```python
from build123d import *

# Parameters (mm, degrees)
F1_DEPTH = 25
F2_DEPTH = 7.5
F3_DEPTH = 12.5
F4_R     = 10
F5_F1_R  = 2
F5_F2_R  = 2
F6_R     = 3.5
F7_DEPTH = 15
F8_R     = 1.99999


# Not quite as in the source:
# - a fillet or chamfer is up to 0.001 mm smaller than in the source, because OpenCascade refuses the exact size


with BuildPart() as f1:
    # F0 (on Top) → F1 (new body, symmetric)
    with BuildSketch(Plane.XY):
        Polygon((-32.5, 5), (-50, 5), (-50, -5), (0, -5), (0, 5), (-17.5, 5), align=None)
    extrude(amount=F1_DEPTH, both=True)

    # F0 (on Top) → F2 (join, symmetric)
    with BuildSketch(Plane.XY):
        with BuildLine():
            Line((-32.5, 28), (-32.5, 5))
            Line((-32.5, 5), (-17.5, 5))
            Line((-17.5, 5), (-17.5, 21))
            ThreePointArc((-17.5, 21), (-14.8639610307, 27.3639610307), (-8.5, 30))
            Line((-8.5, 30), (10, 30))
            Line((10, 30), (10, 37))
            Line((10, 37), (-23.5, 37))
            ThreePointArc((-23.5, 37), (-29.8639610307, 34.3639610307), (-32.5, 28))
        make_face()
    extrude(amount=F2_DEPTH, both=True)

    # F0 (on Top) → F3 (join, symmetric)
    with BuildSketch(Plane.XY):
        Polygon((10, 41), (10, 37), (10, 30), (10, 26), (30, 26), (30, 41), align=None)
    extrude(amount=F3_DEPTH, both=True)

    # F4
    f4_edges = [f1.edges().sort_by_distance(p)[0] for p in [
        (-50, 0, 25),
        (0, 0, 25),
        (0, 0, -25),
        (-50, 0, -25),
    ]]
    fillet(f4_edges, radius=F4_R)

    # F5: fillet of radius 2 on 26 edges, made by hand

    # F5_f1
    f5_f1_edges = [f1.edges().sort_by_distance(p)[0] for p in [
        (0.75, 30, 7.5),
        (-6.75, 37, 7.5),
        (-29.8639610307, 34.3639610307, 7.5),
        (-32.5, 16.5, 7.5),
        (-17.5, 13, 7.5),
        (-14.8639610307, 27.3639610307, 7.5),
        (0.75, 30, -7.5),
        (-6.75, 37, -7.5),
        (-29.8639610307, 34.3639610307, -7.5),
        (-32.5, 16.5, -7.5),
        (-17.5, 13, -7.5),
        (-14.8639610307, 27.3639610307, -7.5),
        (-50, 5, 0),
        (-47.0710678119, 5, -22.0710678119),
        (-47.0710678119, 5, 22.0710678119),
        (-25, 5, -25),
        (-25, 5, 25),
        (-2.9289321881, 5, -22.0710678119),
        (-2.9289321881, 5, 22.0710678119),
        (0, 5, 0),
    ]]
    fillet(f5_f1_edges, radius=F5_F1_R)

    # F5_f2
    f5_f2_edges = [f1.edges().sort_by_distance(p)[0] for p in [
        (10, 33.5, 7.5),
        (-25, 5, 7.5),
        (10, 33.5, -7.5),
        (-25, 5, -7.5),
        (-17.5, 5, 0),
        (-32.5, 5, 0),
        (-31.9142135624, 5, -6.9142135624),
        (-31.9142135624, 5, 6.9142135624),
        (-18.0857864376, 5, 6.9142135624),
        (-18.0857864376, 5, -6.9142135624),
        (10, 30.5857864376, -6.9142135624),
        (10, 36.4142135624, -6.9142135624),
        (10, 30.5857864376, 6.9142135624),
        (10, 36.4142135624, 6.9142135624),
    ]]
    fillet(f5_f2_edges, radius=F5_F2_R)

    # F6 (on face) → F7 (cut, through all)
    with BuildSketch(Plane(origin=(0, 41, 0), x_dir=(-1, 0, 0), z_dir=(0, 1, 0))):
        with Locations((-20, 0)):
            Circle(F6_R)
    extrude(amount=-F7_DEPTH, mode=Mode.SUBTRACT)

    # F8 (radius 2 in the source; OpenCascade refuses exactly that, so slightly less here)
    f8_edges = [f1.edges().sort_by_distance(p)[0] for p in [
        (10, 33.5, -12.5),
        (20, 26, -12.5),
        (30, 33.5, -12.5),
        (20, 41, -12.5),
        (10, 33.5, 12.5),
        (20, 26, 12.5),
        (30, 33.5, 12.5),
        (20, 41, 12.5),
        (30, 41, 0),
        (30, 26, 0),
        (10, 41, 0),
        (10, 26, 0),
    ]]
    fillet(f8_edges, radius=F8_R)


solid = f1.part
```
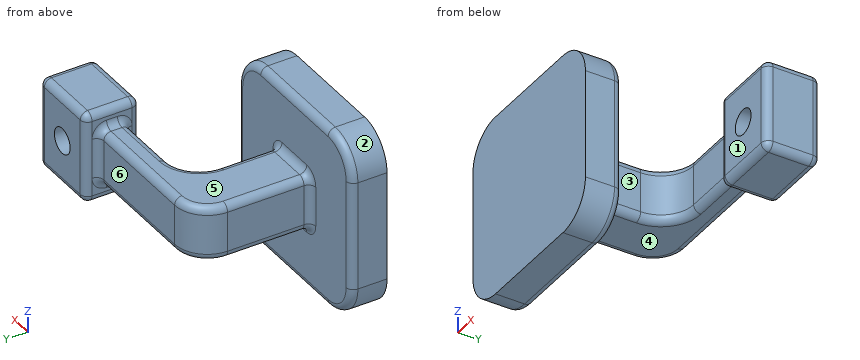
Geometry check sheet. Reference: the model listing, model coordinates, mm. Face numbers are marked on the shaded views. A direction names the side the tool comes from. Coordinates: 2 decimals unless noted, no trailing zeros. Order: outer loops, then holes, each group sorted by start corner. A loop starts at its lowest first (then second) coordinate and runs counter-clockwise, first axis right, second up.
Q1. Draft check along Y on the marked faces 1, 2 and 3. Enter one of: released by +Y, released by -Y, zero draft, split by the parting line, or undercut.
Reply:
face 1: released by -Y
face 2: zero draft
face 3: undercut
Q2. Sectioned sample at D-D on z = 11.5. Record the cut outline in (x, y), and give its area (3 significant figures).
Reply:
outline: (-50, -5) - (0, -5) - (0, 3) arc R2 ccw to (-2, 5) - (-48, 5) arc R2 ccw to (-50, 3) - close; (10.27, 28) arc R1.73 ccw to (12, 26.27) - (28, 26.27) arc R1.73 ccw to (29.73, 28) - (29.73, 39) arc R1.73 ccw to (28, 40.73) - (12, 40.73) arc R1.73 ccw to (10.27, 39) - close
area: 777 mm2
Q3. Depth check by flat-ended pin: pin 1 Ø5 at (x, z) = (17, 8.5) entering from -Y; pin 2 Ø14 at (x, y) = (-20, 25.5) entering from -Z; pin 3 Ø9 at (y, z) = (16, 2) entering from -X; pin 4 Ø8 at (y, z) = (5.5, 2.5) entering from -X. Enter the tip coordinate at first touch or a pass-through.
Reply:
pin 1: stops at y = 26
pin 2: stops at z = -7.5
pin 3: stops at x = -32.5
pin 4: stops at x = -50
Q4. Tool access check on the marked faces 4, 5 and 6. Record the directions out of +Z, -Z, +X, -X, +Y, -Y that give a thin tool (end or side, any length) a straight path to the whole face; none if there is none.
Reply:
face 4: -Z, -X, +Y
face 5: +Z, -X, +Y
face 6: +Z, -Z, -X, +Y
Q5. Sectioned sample at C-C on y = 18. Record the cut outline in (x, z).
Reply:
outline: (-32.5, -5.5) arc R2 ccw to (-30.5, -7.5) - (-19.5, -7.5) arc R2 ccw to (-17.5, -5.5) - (-17.5, 5.5) arc R2 ccw to (-19.5, 7.5) - (-30.5, 7.5) arc R2 ccw to (-32.5, 5.5) - close
Q6. Thickness scan on probe 1 along Z at (x, y) = (20, 32); probe 2 along Y at (x, z) = (-19, 20); probe 3 along Y at (x, z) = (-14.5, 6). Record the ranges inside material, lowest first.
Reply:
probe 1: z = -12.5 to -3.5, 3.5 to 12.5
probe 2: y = -5 to 5
probe 3: y = -5 to 5, 27.79 to 36.94
Q7. Sectioned sample at A-A on x = 20. Record the cut outline in (y, z).
Reply:
outline: (26, -10.5) arc R2 ccw to (28, -12.5) - (39, -12.5) arc R2 ccw to (41, -10.5) - (41, -3.5) - (26, -3.5) - close; (26, 3.5) - (41, 3.5) - (41, 10.5) arc R2 ccw to (39, 12.5) - (28, 12.5) arc R2 ccw to (26, 10.5) - close
